The listing builds one solid part. Answer for the finished solid, in the listing's coordinates (mm). Give positions to 0.01 mm unless a question says otherwise; leave off trailing zeros. Loops run counter-clockwise (first coordinate to the right, second up) from the corner with the lowest first, then second, coordinate; pieces in that order, holes last. Notation, with made-up numbers: M 80,51 L 105,51 A26 ccw 105,89 Z; hole C -2,2.5 d9. An arc over 180 degrees is marked long. One line per item, written item: value. Start each with the question number.
Q1. A cutting plane is placed at B-B, the plane y = 1.5. Determine the outline of the cut face in (x, z), and give its area (3 significant figures).
Q2. A cutting plane is placed at A-A, the plane z = 1.35. Determine the outline of the cut face in (x, y).
Q3. Consider L1, parallel to Y at x = -1, z = 0.35; L2, parallel to Y at x = 69.5, z = 0.6; L3, parallel to X at y = 90, z = 0.7. Determine where each line is inside the solid, lowest interval first.
Q4. Flat-ended cylindrical pins translate along their axes: pin 1 (2 mm diameter, centred on x = 7.35, y = 133.6, fed in from -Z); pin 2 (3 mm diameter, centred on x = 76.93, y = 64.01, fed in from -Z); pin 3 (1 mm diameter, centred on x = -64.5, z = 1, fed in from -Y). Find the tip coordinate at first contact, or state that the pin passes through.
Q5. A cutting plane is placed at C-C, the plane x = -28. Determine the outline of the cut face in (y, z), and give its area (3 significant figures).
from build123d import *

# Parameters (mm, degrees)
ESBO_O1_R                = 1.25
RESSALTO_EXTRUS_O1_DEPTH = 2


with BuildPart() as part:
    # Esboço1 → Ressalto-extrusão1 (new body)
    with BuildSketch(Plane.XY):
        with BuildLine():
            Line((64.019528598, 84.846815111), (84.16137873, 64.704964979))
            ThreePointArc((84.16137873, 64.704964979), (49.309954929, -12.012204688), (-34.522641382, -20.511713992))
            Line((-34.522641382, -20.511713992), (-76.621548101, 20.929016434))
            ThreePointArc((-76.621548101, 20.929016434), (-69.061916809, 105.430734899), (8.041603414, 140.824740295))
            Line((8.041603414, 140.824740295), (28.423773233, 120.442570476))
            Line((28.423773233, 120.442570476), (64.019528598, 84.846815111))
        make_face()
        with Locations((-31.557799421, -13.88383463)):
            Circle(ESBO_O1_R, mode=Mode.SUBTRACT)
        with Locations((7.350981773, 133.596869623)):
            Circle(ESBO_O1_R, mode=Mode.SUBTRACT)
        with Locations((76.933508058, 64.014343338)):
            Circle(ESBO_O1_R, mode=Mode.SUBTRACT)
        with Locations((-70.041206278, 23.99792083)):
            Circle(ESBO_O1_R, mode=Mode.SUBTRACT)
    extrude(amount=RESSALTO_EXTRUS_O1_DEPTH)


solid = part.part
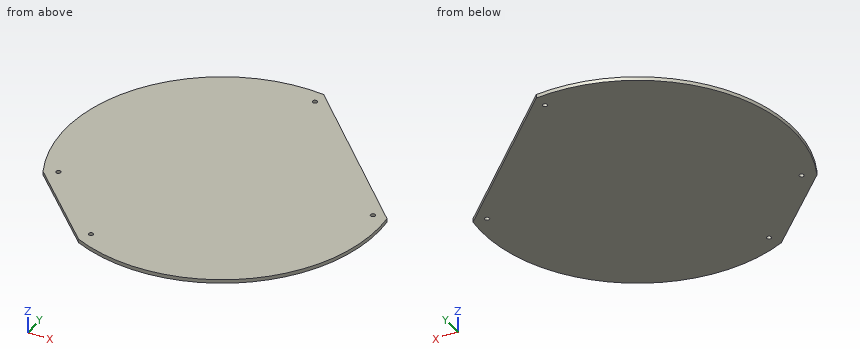
Answer block:
1. outline: M -56.88,0 L 64.07,0 L 64.07,2 L -56.88,2 Z
1. area: 242 mm^2
2. outline: M -76.62,20.93 L -34.52,-20.51 A84.54 ccw 84.16,64.7 L 8.04,140.82 A84.54 ccw Z; hole C -70.04,24 d2.5; hole C -31.56,-13.88 d2.5; hole C 7.35,133.6 d2.5; hole C 76.93,64.01 d2.5
3. L1: -27.88 to 141.2
3. L2: 8.52 to 79.37
3. L3: -77.69 to 58.87
4. pin 1: through
4. pin 2: z = 0
4. pin 3: y = 8.5
5. outline: M -23.11,0 L 136.44,0 L 136.44,2 L -23.11,2 Z
5. area: 319 mm^2
